from build123d import *

# Parameters (mm, degrees)
ESQUISSE1_W        = 71.5
ESQUISSE1_H        = 39.2
BOSS_EXTRU_1_DEPTH = 24
ESQUISSE2_W        = 79.3
ESQUISSE2_H        = 43.2
BOSS_EXTRU_2_DEPTH = 2
ESQUISSE3_R        = 6.4
BOSS_EXTRU_3_DEPTH = 11.7


with BuildPart() as part:
    # Esquisse1 → Boss.-Extru.1 (new body)
    with BuildSketch(Plane.XY):
        with Locations((35.75, -19.6)):
            Rectangle(ESQUISSE1_W, ESQUISSE1_H)
    extrude(amount=BOSS_EXTRU_1_DEPTH)

    # Esquisse2 → Boss.-Extru.2 (add)
    with BuildSketch(Plane.XY.offset(24)):
        with Locations((35.75, -19.6)):
            Rectangle(ESQUISSE2_W, ESQUISSE2_H)
    extrude(amount=BOSS_EXTRU_2_DEPTH)

    # Esquisse3 → Boss.-Extru.3 (add)
    with BuildSketch(Plane.XY.offset(26)):
        with Locations((55.105708791, -14.4)):
            Circle(ESQUISSE3_R)
    extrude(amount=BOSS_EXTRU_3_DEPTH)


solid = part.part
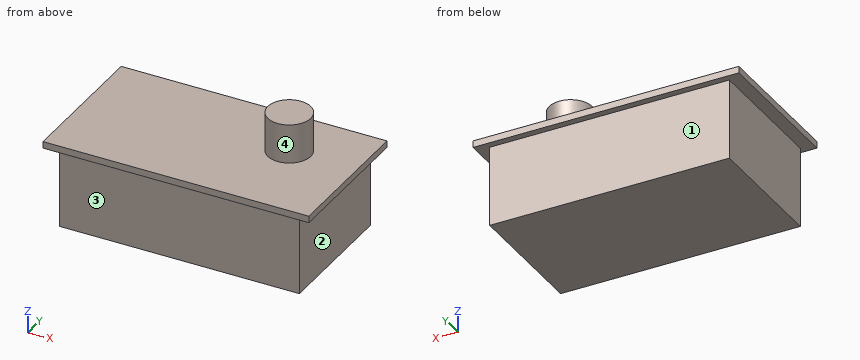
Read the model definition and answer for the solid it produces. Units are mm, in the model's axes. Face numbers are marked on the shaded views. A direction names the side the tool comes from. Coordinates: 2 decimals unless noted, no trailing zeros. Order: outer loops, then holes, each group sorted by start corner. A loop starts at its lowest first (then second) coordinate and runs counter-clockwise, first axis right, second up. Notation, with made-up numbers: M 66.5,52.5 L 105.5,52.5 A34 cw 105.5,90.5 Z; hole C 1.5,-35.75 d6. An arc over 180 degrees is marked long. Put each result on its own line as item: value. Start each with the question number.
Item 1: Section B-B, the plane x = 15.5 is taken. Determine the outline of the cut face in (y, z).
Item 2: Section A-A, the plane y = -5.5 is taken. Determine the outline of the cut face in (x, z).
Item 3: Given pin 1 Ø12 at (y, z) = (-22, 16) entering from -X; pin 2 Ø5 at (y, z) = (-8, 16.5) entering from +X; pin 3 Ø21.5 at (x, y) = (16.5, -10.5) entering from +Z, each flat-ended and moving along its own axis, determine where each tip first touches the part or whether it passes through.
Item 4: Section D-D, the plane y = -14.4 is taken. Determine the outline of the cut face in (x, z), plus the area to 3 significant figures.
Item 5: For the marked faces 1, 2, 3 and 4, determine the directions among +Z, -Z, +X, -X, +Y, -Y from which every point of the face is accessible in a straight line to the end or side of a thin tool.
Item 6: Consider probe 1 along X at (y, z) = (-12, 21); probe 2 along Z at (x, y) = (67, -15); probe 3 along Y at (x, z) = (58.5, 2). Determine where each line is inside the solid, lowest interval first. Write a range as [from, to].
Item 7: Section C-C, the plane z = 9.5 is taken. Determine the outline of the cut face in (x, y), plus the area to 3 significant figures.
Computed:
1. outline: M -41.2,24 L -39.2,24 L -39.2,0 L 0,0 L 0,24 L 2,24 L 2,26 L -41.2,26 Z
2. outline: M -3.9,24 L 0,24 L 0,0 L 71.5,0 L 71.5,24 L 75.4,24 L 75.4,26 L -3.9,26 Z
3. pin 1: stops at x = 0
3. pin 2: stops at x = 71.5
3. pin 3: stops at z = 26
4. outline: M -3.9,24 L 0,24 L 0,0 L 71.5,0 L 71.5,24 L 75.4,24 L 75.4,26 L 61.51,26 L 61.51,37.7 L 48.71,37.7 L 48.71,26 L -3.9,26 Z
4. area: 2,020 mm2
5. face 1: -Z, +X, -X, +Y
5. face 2: -Z, +X, +Y, -Y
5. face 3: -Z, +X, -X, -Y
5. face 4: +Z
6. probe 1: x = [0, 71.5]
6. probe 2: z = [0, 26]
6. probe 3: y = [-39.2, 0]
7. outline: M 0,-39.2 L 71.5,-39.2 L 71.5,0 L 0,0 Z
7. area: 2,800 mm2
